Geometry: final body of the model. Coordinates: model frame, mm. A direction names the side the tool comes from. Coordinates: 2 decimals unless noted, no trailing zeros. Order: outer loops, then holes, each group sorted by start corner. A loop starts at its lowest first (then second) coordinate and runs counter-clockwise, first axis right, second up. Notation, with made-up numbers: (25, 8.5) -> (49, 8.5) arc R25 ccw to (49, 22.5) -> close; hole circle Ø4 at (27, 24). An arc over 180 degrees is marked (long way). Answer in a Markdown table with one row per item. Add a question column.
1) Section query A-A on z = 10. Return the cut outline in (x, y).
2) Section query B-B on x = 17. Return the cut outline in (y, z), then the cut area to 3 significant figures.
3) Section query C-C on z = 22.5. Return the cut outline in (x, y).
4) Section query D-D on y = 19. Return the cut outline in (x, z), then the cut area to 3 significant figures.
5) Contact query for flat-ended pins moving along their axis: P1, Ø1.5, axis at y = -5.5, z = 18, coming from the +X side; P2, Ø6.5, axis at x = 12.5, y = 12.5, coming from the -Z side; P3, Ø1, axis at x = 13.5, z = 9.5, coming from the -Y side. Output: stop coordinate, or through.
6) Ray query, line 1 (Y direction, x = 12, z = 2); line 2 (Z direction, x = -9, y = 12); line 3 (Z direction, x = -16.5, y = -7). Return the intervals inside material, ascending. Write a range as from..to.
7) Pull-direction query (Y, two-part tool) for faces 5 (the face through (6.55, -4.96, 21.45)), 6 (the face through (9.18, -8.41, -5.18)), 7 (the face through (8.16, -5.31, 3.21)), 8 (the face through (0, 0, 24.8)); classes: +Y half, -Y half, draft (parallel to the pull), parting line (faces both ways), or undercut.
8) Set-up query: faces 1 (the face through (11.464, -16.768, 14.94)), 2 (the face through (16.723, -11.42, 14.94)), 3 (the face through (-11.42, -16.723, 14.94)), 4 (the face through (-9.9, -9.8, 14.7)). Return all of +Z, -Z, +X, -X, +Y, -Y with unobstructed straight access to the full face (end or side cutting, diameter ignored); none if empty.
Autodesk Inventor part; units mm, degrees
ref_plane "YZ Plane" through (0, 0, 0) normal (1, 0, 0) x (0, 1, 0)
ref_plane "XZ Plane" through (0, 0, 0) normal (0, 1, 0) x (-1, 0, 0)
ref_plane "XY Plane" through (0, 0, 0) normal (0, 0, 1) x (1, 0, 0)
sketch "Sketch1" plane through (0, 0, 0) normal (0, 0, 1) x (1, 0, 0)
  circle A0 centre (0, 0) radius 22.5
  dimension "d0" = 45
extrude "Extrusion1" add sketch "Sketch1" along normal blind 24.8
sketch "Sketch2" plane through (0, 0, 0) normal (0, 0, -1) x (-1, 0, 0)
  circle A0 centre (0, 0) radius 12.45
  dimension "d3" = 24.9
extrude "Extrusion2" add sketch "Sketch2" along normal blind 12
sketch "Sketch3" plane through (0, 0, 24.8) normal (0, 0, 1) x (1, 0, 0)
  line L0 (12.5, -12.5) -> (-12.5, -12.5) construction
  line L1 (-12.5, -12.5) -> (-12.5, 12.5) construction
  line L2 (-12.5, 12.5) -> (12.5, 12.5) construction
  line L3 (12.5, 12.5) -> (12.5, -12.5) construction
  line L4 (12.5, -12.5) -> (-12.5, 12.5) construction
  line L5 (-12.5, -12.5) -> (12.5, 12.5) construction
  point P0 (0, 0)
  dimension "d6" = 25
  dimension "d7" = 25
hole "Hole1" at (-12.5, 12.5, 24.8) at (12.5, 12.5, 24.8) at (12.5, -12.5, 24.8) at (-12.5, -12.5, 24.8) direction (0, 0, -1) diameter 4.2 end through all counterbore diameter 7.5 counterbore depth 20
sketch "Sketch4" plane through (0, 0, 24.8) normal (0, 0, 1) x (1, 0, 0)
  line L0 (-13.2583, 18.5616) -> (-9.8483, 15.1517)
  line L1 (-9.8483, 15.1517) -> (-15.1517, 9.8483)
  line L2 (-15.1517, 9.8483) -> (-18.5616, 13.2583)
  line L3 (-18.5616, 13.2583) -> (-13.2583, 18.5616)
  line L4 (-13.2583, 18.5616) -> (-15.1517, 9.8483) construction
  line L5 (-9.8483, 15.1517) -> (-18.5616, 13.2583) construction
  circle A0 centre (-12.5, 12.5) radius 3.75
  circle A1 centre (0, 0) radius 22.5
  circle A2 centre (-12.5, 12.5) radius 3.75 construction
  line L6 (-14.205, 14.205) -> (-12.5, 12.5) construction
  point P0 (-18.339, 13.0357)
  point P1 (-13.0357, 18.339)
extrude "Extrusion3" cut sketch "Sketch4" against normal up to surface (20 mm away) contours L0 A0 L2 A1 | L1 A0 picked at (-13.4167, 17.3703) picked at (-13.3264, 14.7238)
pattern_circular "Circular Pattern1" count 4 over 360 about axis through (0, 0, 0) along (0, 0, 1) of "Extrusion3"
chamfer "Chamfer1" distance 1.5 angle 45 1 edges at (12.45, 0, -12)
sketch "Sketch5" plane through (0, 0, -12) normal (0, 0, -1) x (-1, 0, 0)
  line L0 (0, 12) -> (-12, 12) construction
  line L1 (-12, 12) -> (-12, -32.1468) construction
  line L2 (-12, -32.1468) -> (0, -32.1468) construction
  line L3 (0, -32.1468) -> (0, 12) construction
  circle A0 centre (-4.5, 4.5) radius 3.75 construction
  circle A1 centre (-4.5, -4.5) radius 3.75 construction
  line L4 (-4.5, -4.5) -> (-4.5, 4.5) construction
  circle A2 centre (0, 0) radius 10.95 construction
  line L5 (31.5, 0) -> (-31.5, 0) construction
  dimension "d23" = 12
  dimension "d24" = 12
  dimension "d25" = 7.5
  dimension "d29" = 9
  dimension "d30" = 4.5
hole "Hole2" at (4.5, -4.5, -12) at (4.5, 4.5, -12) direction (0, 0, 1) diameter 4.2 end through all counterbore diameter 7.5 counterbore depth 30
properties part number "StageConnection" material "Aluminum 6061"
Result:
| question | item | result |
|---|---|---|
| 1 | outline | (-18.34, -13.04) -> (-15.15, -9.85) arc R3.75 cw to (-9.85, -15.15) -> (-13.04, -18.34) arc R22.5 ccw to (13.04, -18.34) -> (9.85, -15.15) arc R3.75 cw to (15.15, -9.85) -> (18.34, -13.04) arc R22.5 ccw to (18.34, 13.04) -> (15.15, 9.85) arc R3.75 cw to (9.85, 15.15) -> (13.04, 18.34) arc R22.5 ccw to (-13.04, 18.34) -> (-9.85, 15.15) arc R3.75 cw to (-15.15, 9.85) -> (-18.34, 13.04) arc R22.5 ccw to start; hole circle Ø7.5 at (4.5, -4.5); hole circle Ø7.5 at (4.5, 4.5) |
| 2 | outline | (-14.74, 0) -> (14.74, 0) -> (14.74, 4.8) -> (11.7, 4.8) -> (11.7, 24.8) -> (-11.7, 24.8) -> (-11.7, 4.8) -> (-14.74, 4.8) -> close |
| 2 | area | 609 mm2 |
| 3 | outline | (-18.34, -13.04) -> (-15.15, -9.85) arc R3.75 cw to (-9.85, -15.15) -> (-13.04, -18.34) arc R22.5 ccw to (13.04, -18.34) -> (9.85, -15.15) arc R3.75 cw to (15.15, -9.85) -> (18.34, -13.04) arc R22.5 ccw to (18.34, 13.04) -> (15.15, 9.85) arc R3.75 cw to (9.85, 15.15) -> (13.04, 18.34) arc R22.5 ccw to (-13.04, 18.34) -> (-9.85, 15.15) arc R3.75 cw to (-15.15, 9.85) -> (-18.34, 13.04) arc R22.5 ccw to start; hole circle Ø4.2 at (4.5, -4.5); hole circle Ø4.2 at (4.5, 4.5) |
| 4 | outline | (-12.05, 0) -> (12.05, 0) -> (12.05, 24.8) -> (-12.05, 24.8) -> close |
| 4 | area | 598 mm2 |
| 5 | P1 | x = 21.99 |
| 5 | P2 | z = 0 |
| 5 | P3 | y = -18.36 |
| 6 | line 1 | -19.03..-14.54, -10.46..10.46, 14.54..19.03 |
| 6 | line 2 | 0..4.8 |
| 6 | line 3 | 0..24.8 |
| 7 | face 5 | undercut |
| 7 | face 6 | parting line |
| 7 | face 7 | undercut |
| 7 | face 8 | draft |
| 8 | face 1 | +Z, +X |
| 8 | face 2 | +Z, -Y |
| 8 | face 3 | +Z, -X |
| 8 | face 4 | +Z |
